from build123d import *

# Parameters (mm, degrees)
SKETCH_R     = 5.75
SKETCH_R_2   = 2
SKETCH_R_3   = 3.25
PAD_DEPTH    = 4
PAD001_DEPTH = 10
SKETCH002_R  = 3
POCKET_DEPTH = 2
FILLET_R     = 1


with BuildPart() as part:
    # Sketch → Pad (new body)
    with BuildSketch(Plane.XY):
        with BuildLine():
            ThreePointArc((-95, 50), (-98.535534, 48.535534), (-100, 45))
            Line((-100, -45), (-100, 45))
            ThreePointArc((-100, -45), (-98.535534, -48.535534), (-95, -50))
            Line((95, -50), (-95, -50))
            ThreePointArc((95, -50), (98.535534, -48.535534), (100, -45))
            Line((100, 45), (100, -45))
            ThreePointArc((100, 45), (98.535534, 48.535534), (95, 50))
            Line((-95, 50), (95, 50))
        make_face()
        Circle(SKETCH_R, mode=Mode.SUBTRACT)
        with Locations((95, 45)):
            Circle(SKETCH_R_2, mode=Mode.SUBTRACT)
        with Locations((95, -45)):
            Circle(SKETCH_R_2, mode=Mode.SUBTRACT)
        with Locations((-95, 45)):
            Circle(SKETCH_R_2, mode=Mode.SUBTRACT)
        with Locations((0, 45)):
            Circle(SKETCH_R_2, mode=Mode.SUBTRACT)
        with Locations((0, -45)):
            Circle(SKETCH_R_2, mode=Mode.SUBTRACT)
        with Locations((30, 20)):
            Circle(SKETCH_R_3, mode=Mode.SUBTRACT)
        with Locations((70, 20)):
            Circle(SKETCH_R_3, mode=Mode.SUBTRACT)
        with Locations((30, -20)):
            Circle(SKETCH_R_3, mode=Mode.SUBTRACT)
        with Locations((70, -20)):
            Circle(SKETCH_R_3, mode=Mode.SUBTRACT)
        with Locations((-53.5, 20)):
            Circle(SKETCH_R_2, mode=Mode.SUBTRACT)
        with Locations((-53.5, -20)):
            Circle(SKETCH_R_2, mode=Mode.SUBTRACT)
        with Locations((-95, -45)):
            Circle(SKETCH_R_2, mode=Mode.SUBTRACT)
        with BuildLine():
            ThreePointArc((-75, 14), (-76.414214, 13.414214), (-77, 12))
            Line((-77, -12), (-77, 12))
            ThreePointArc((-77, -12), (-76.414214, -13.414214), (-75, -14))
            Line((-32, -14), (-75, -14))
            ThreePointArc((-32, -14), (-30.585786, -13.414214), (-30, -12))
            Line((-30, 12), (-30, -12))
            ThreePointArc((-30, 12), (-30.585786, 13.414214), (-32, 14))
            Line((-75, 14), (-32, 14))
        make_face(mode=Mode.SUBTRACT)
    extrude(amount=PAD_DEPTH)

    # Sketch001 (on Face31 of Pad) → Pad001 (join)
    with BuildSketch(Plane.XY.offset(4)):
        with BuildLine():
            ThreePointArc((-82.5, 36.5), (-89.571068, 33.571068), (-92.5, 26.5))
            Line((-92.5, -26.5), (-92.5, 26.5))
            ThreePointArc((-92.5, -26.5), (-89.571068, -33.571068), (-82.5, -36.5))
            Line((82.5, -36.5), (-82.5, -36.5))
            ThreePointArc((82.5, -36.5), (89.571068, -33.571068), (92.5, -26.5))
            Line((92.5, 26.5), (92.5, -26.5))
            ThreePointArc((92.5, 26.5), (89.571068, 33.571068), (82.5, 36.5))
            Line((-82.5, 36.5), (82.5, 36.5))
        make_face()
        with BuildLine():
            ThreePointArc((-82.5, 34.5), (-88.156854, 32.156854), (-90.5, 26.5))
            Line((-90.5, -26.5), (-90.5, 26.5))
            ThreePointArc((-90.5, -26.5), (-88.156854, -32.156854), (-82.5, -34.5))
            Line((82.5, -34.5), (-82.5, -34.5))
            ThreePointArc((82.5, -34.5), (88.156854, -32.156854), (90.5, -26.5))
            Line((90.5, 26.5), (90.5, -26.5))
            ThreePointArc((90.5, 26.5), (88.156854, 32.156854), (82.5, 34.5))
            Line((-82.5, 34.5), (82.5, 34.5))
        make_face(mode=Mode.SUBTRACT)
    extrude(amount=PAD001_DEPTH)

    # Sketch002 (on Face4 of Pad001) → Pocket (cut)
    with BuildSketch(Plane(origin=(0, 0, 0), x_dir=(1, 0, 0), z_dir=(0, 0, -1))):
        with Locations((-95, 45)):
            Circle(SKETCH002_R)
        with Locations((0, 45)):
            Circle(SKETCH002_R)
        with Locations((95, 45)):
            Circle(SKETCH002_R)
        with Locations((95, -45)):
            Circle(SKETCH002_R)
        with Locations((0, -45)):
            Circle(SKETCH002_R)
        with Locations((-95, -45)):
            Circle(SKETCH002_R)
    extrude(amount=-POCKET_DEPTH, mode=Mode.SUBTRACT)

    # Fillet
    fillet_edges = [part.edges().sort_by_distance(p)[0] for p in [
        (0, -50, 0),
    ]]
    fillet(fillet_edges, radius=FILLET_R)


solid = part.part
The model under review builds one solid part; all positions refer to its coordinate system, in mm. A direction names the side the tool comes from. Round coordinates to 2 decimals unless told otherwise and drop trailing zeros. Loops run counter-clockwise (first coordinate to the right, second up) from the corner with the lowest first, then second, coordinate; pieces in that order, holes last. Notation, with made-up numbers: (45, 42.5) -> (94, 42.5) arc R37 ccw to (94, 78.5) -> close; hole circle Ø4 at (-40, 32.25). An arc over 180 degrees is marked (long way). One line per question, with ' | ' between items. Start each with the question number.
Item 1: Wall thickness on line 1 along Y through (x, z) = (95, 3.5); line 2 along X through (y, z) = (-45, 1.1); line 3 along X through (y, z) = (45, 3.3): over which ranges is each line inside the solid? List them lowest first. Write a range as [from, to].
Item 2: For pin 1 (8 mm diameter, centred on y = 13, z = 12, fed in from -X); pin 2 (8 mm diameter, centred on x = 0, y = 45, fed in from +Z); pin 3 (4.5 mm diameter, centred on x = 0, y = 45, fed in from -Z), all flat-tipped, find the tip position at first contact; note any pin that passes through.
Item 3: Add section C-C, the plane y = 0. Write out the cut boundary in (x, z).
Item 4: Add section D-D, the plane x = 0. Count the separate pieces of the cut face and the enclosed holes in it, then the cut area to 3 significant figures.
Item 5: Add section B-B, the plane x = -42. Write out the cut boundary in (y, z).
Item 6: Draft analysis for pull direction X (two halves, no side actions). For faces 4 (the face through (-89.49, 33.65, 8.93)), 5 (the face through (-8, -37, 4)), 6 (the face through (92, 45, 1)), state which applies: +X half, -X half, draft (parallel to the pull), parting line (faces both ways), or undercut.
Item 7: Machinability: for faces 1 (the face through (90.5, 0, 9)), 2 (the face through (1, -36.5, 9)), 3 (the face through (-94, 47, 2)), which of the approach directions +Z, -Z, +X, -X, +Y, -Y give a long, thin tool a straight path to every point of the face, cutting with its end or side? Answer none if there is none.
Item 8: Add section A-A, the plane y = -20. Write out the cut boundary in (x, z), then the cut area to 3 significant figures.
Return value:
1) line 1: y = [-50, -47], [-43, 43], [47, 50] | line 2: x = [-100, -98], [-92, -3], [3, 92], [98, 100] | line 3: x = [-100, -97], [-93, -2], [2, 93], [97, 100]
2) pin 1: stops at x = -92.5 | pin 2: stops at z = 4 | pin 3: stops at z = 2
3) outline: (-100, 1) arc R1 ccw to (-99, 0) -> (-77, 0) -> (-77, 4) -> (-90.5, 4) -> (-90.5, 14) -> (-92.5, 14) -> (-92.5, 4) -> (-100, 4) -> close; (-30, 0) -> (-5.75, 0) -> (-5.75, 4) -> (-30, 4) -> close; (5.75, 0) -> (99, 0) arc R1 ccw to (100, 1) -> (100, 4) -> (92.5, 4) -> (92.5, 14) -> (90.5, 14) -> (90.5, 4) -> (5.75, 4) -> close
4) separate pieces: 4 | enclosed holes: 0 | area: 354 mm2
5) outline: (-50, 1) arc R1 ccw to (-49, 0) -> (-14, 0) -> (-14, 4) -> (-34.5, 4) -> (-34.5, 14) -> (-36.5, 14) -> (-36.5, 4) -> (-50, 4) -> close; (14, 0) -> (49, 0) arc R1 ccw to (50, 1) -> (50, 4) -> (36.5, 4) -> (36.5, 14) -> (34.5, 14) -> (34.5, 4) -> (14, 4) -> close
6) face 4: -X half | face 5: draft | face 6: undercut
7) face 1: +Z | face 2: +Z, +X, -X, -Y | face 3: -Z
8) outline: (-100, 1) arc R1 ccw to (-99, 0) -> (-55.5, 0) -> (-55.5, 4) -> (-90.5, 4) -> (-90.5, 14) -> (-92.5, 14) -> (-92.5, 4) -> (-100, 4) -> close; (-51.5, 0) -> (26.75, 0) -> (26.75, 4) -> (-51.5, 4) -> close; (33.25, 0) -> (66.75, 0) -> (66.75, 4) -> (33.25, 4) -> close; (73.25, 0) -> (99, 0) arc R1 ccw to (100, 1) -> (100, 4) -> (92.5, 4) -> (92.5, 14) -> (90.5, 14) -> (90.5, 4) -> (73.25, 4) -> close | area: 772 mm2
